from build123d import *

# Parameters (mm, degrees)
SKETCH_1_R          = 17.5
SKETCH_1_R_2        = 1.65
SKETCH_1_R_3        = 1.75
EXTRUDE_1_DEPTH     = 7
SKETCH_2_R          = 2.9
CUT_EXTRUDE_1_DEPTH = 3


with BuildPart() as part:
    # 草图1 → 凸台-拉伸1 (new body)
    with BuildSketch(Plane(origin=(0, 0, 0), x_dir=(1, 0, 0), z_dir=(0, 1, 0))):
        with Locations(Location((0, 0, 0), (0, 0, 270))):
            Circle(SKETCH_1_R)
        with Locations(Location((-14, 0, 0), (0, 0, 270))):
            Circle(SKETCH_1_R_2, mode=Mode.SUBTRACT)
        with Locations(Location((-7, 12.124355653, 0), (0, 0, 270))):
            Circle(SKETCH_1_R_2, mode=Mode.SUBTRACT)
        with Locations(Location((7, 12.124355653, 0), (0, 0, 270))):
            Circle(SKETCH_1_R_2, mode=Mode.SUBTRACT)
        with Locations(Location((14, 0, 0), (0, 0, 270))):
            Circle(SKETCH_1_R_2, mode=Mode.SUBTRACT)
        with Locations(Location((7, -12.124355653, 0), (0, 0, 270))):
            Circle(SKETCH_1_R_2, mode=Mode.SUBTRACT)
        with Locations(Location((-7, -12.124355653, 0), (0, 0, 270))):
            Circle(SKETCH_1_R_2, mode=Mode.SUBTRACT)
        with Locations(Location((0, 0, 0), (0, 0, 270))):
            Circle(SKETCH_1_R_3, mode=Mode.SUBTRACT)
        with Locations(Location((7, 0, 0), (0, 0, 270))):
            Circle(SKETCH_1_R_2, mode=Mode.SUBTRACT)
        with Locations(Location((0, -7, 0), (0, 0, 270))):
            Circle(SKETCH_1_R_2, mode=Mode.SUBTRACT)
        with Locations(Location((-7, 0, 0), (0, 0, 270))):
            Circle(SKETCH_1_R_2, mode=Mode.SUBTRACT)
        with Locations(Location((0, 7, 0), (0, 0, 270))):
            Circle(SKETCH_1_R_2, mode=Mode.SUBTRACT)
    extrude(amount=EXTRUDE_1_DEPTH)

    # 草图2 → 切除-拉伸1 (cut)
    with BuildSketch(Plane(origin=(0, 7, 0), x_dir=(1, 0, 0), z_dir=(0, 1, 0))):
        with Locations(Location((-14, 0, 0), (0, 0, 270))):
            Circle(SKETCH_2_R)
        with Locations(Location((-7, 12.124355653, 0), (0, 0, 270))):
            Circle(SKETCH_2_R)
        with Locations(Location((7, 12.124355653, 0), (0, 0, 270))):
            Circle(SKETCH_2_R)
        with Locations(Location((14, 0, 0), (0, 0, 270))):
            Circle(SKETCH_2_R)
        with Locations(Location((7, -12.124355653, 0), (0, 0, 270))):
            Circle(SKETCH_2_R)
        with Locations(Location((-7, -12.124355653, 0), (0, 0, 270))):
            Circle(SKETCH_2_R)
    extrude(amount=-CUT_EXTRUDE_1_DEPTH, mode=Mode.SUBTRACT)


solid = part.part
The model under review builds one solid part; all positions refer to its coordinate system, in mm. A direction names the side the tool comes from. Coordinates: 2 decimals unless noted, no trailing zeros. Loops run counter-clockwise (first coordinate to the right, second up) from the corner with the lowest first, then second, coordinate; pieces in that order, holes last. Notation, with made-up numbers: (79.5, -23.5) -> (134.5, -23.5) arc R15 cw to (134.5, -19.5) -> close; hole circle Ø4 at (68.5, 50.5). An arc over 180 degrees is marked (long way). Use a Markdown table: item, result. Add a question column.
1. Machinability: for faces 3 (the face through (-7, 4, -10)), 4 (the face through (0.07, 3.45, -8.65)), which of the approach directions +Z, -Z, +X, -X, +Y, -Y give a long, thin tool a straight path to every point of the face, cutting with its end or side? Answer none if there is none.
2. Add section B-B on x = 14. Write out the cut boundary in (y, z).
3. Add section D-D on z = 7. Write out the cut boundary in (x, y).
4. Clearance check with flat-ended pins moving along their axes: pin 1 Ø4 at (x, z) = (7, -12.12) entering from +Y; pin 2 Ø2.5 at (x, z) = (7, 0) entering from -Y. State where each tip first meets the part, or that it passes through.
5. Draft analysis for pull direction X (two halves, no side actions). For faces 1 (the face through (-10.648, 3.451, -13.887)), 2 (the face through (11.17, 5.52, -0.63)), state which applies: pulls with the +X half, pulls with the -X half, needs draft (parallel to the pull), parting line crosses it, or undercut.
6. To check wall thickness, follow line 1 (X direction, y = 3, z = 0); line 2 (X direction, y = 6.5, z = -1.5); line 3 (Z direction, x = 4.5, y = 6.5). State the ranges of each line that lie inside material, in increasing order.
7. Add section A-A on z = 0. Give the number of separate pieces and of enclosed holes in the cut face, plus the area to 3 significant figures.
Returned:
| question | item | result |
|---|---|---|
| 1 | face 3 | +Y |
| 1 | face 4 | +Y, -Y |
| 2 | outline | (0, -10.5) -> (7, -10.5) -> (7, -2.9) -> (4, -2.9) -> (4, -1.65) -> (0, -1.65) -> close; (0, 1.65) -> (4, 1.65) -> (4, 2.9) -> (7, 2.9) -> (7, 10.5) -> (0, 10.5) -> close |
| 3 | outline | (-16.04, 0) -> (-1.65, 0) -> (-1.65, 7) -> (-16.04, 7) -> close; (1.65, 0) -> (16.04, 0) -> (16.04, 7) -> (1.65, 7) -> close |
| 4 | pin 1 | stops at y = 4 |
| 4 | pin 2 | passes through |
| 5 | face 1 | parting line crosses it |
| 5 | face 2 | undercut |
| 6 | line 1 | x = -17.5 to -15.65, -12.35 to -8.65, -5.35 to -1.75, 1.75 to 5.35, 8.65 to 12.35, 15.65 to 17.5 |
| 6 | line 2 | x = -17.44 to -16.48, -11.52 to -7.69, -6.31 to -0.9, 0.9 to 6.31, 7.69 to 11.52, 16.48 to 17.44 |
| 6 | line 3 | z = -16.91 to -13.59, -10.65 to 10.65, 13.59 to 16.91 |
| 7 | separate pieces | 6 |
| 7 | enclosed holes | 0 |
| 7 | area | 113 mm² |
